Check sheet for the modelled part. Datum: model origin and axes. Units: mm. Face numbers are marked on the shaded views. A direction names the side the tool comes from. Round coordinates to 2 decimals unless told otherwise and drop trailing zeros. Write each loop counter-clockwise with the first axis right and the second up, starting at its lowest first coordinate (ties: lowest second). Pieces come first, ordered by that corner, then holes. Notation, with made-up numbers: (2, -14.5) -> (46, -14.5) arc R24 ccw to (46, 12.5) -> close; hole circle Ø5 at (66.25, 72.5). An arc over 180 degrees is marked (long way). One line per item, written item: value.
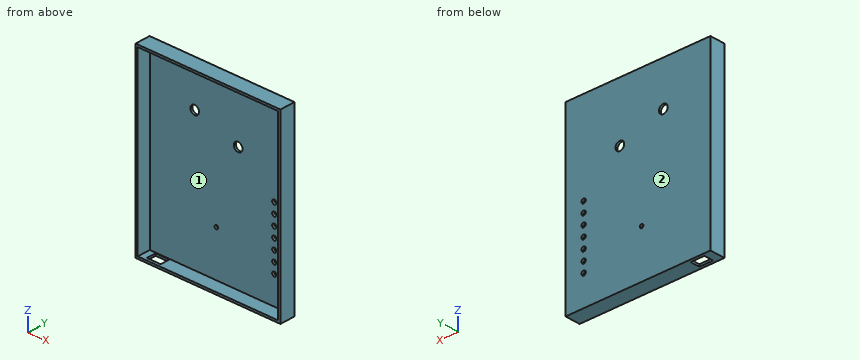
Autodesk Inventor part; units mm, degrees
ref_plane "YZ Plane" through (0, 0, 0) normal (1, 0, 0) x (0, 1, 0)
ref_plane "XZ Plane" through (0, 0, 0) normal (0, 1, 0) x (-1, 0, 0)
ref_plane "XY Plane" through (0, 0, 0) normal (0, 0, 1) x (1, 0, 0)
sketch "block" plane through (0, 0, 0) normal (0, 1, 0) x (-1, 0, 0)
  line L0 (0, 0) -> (-200, 0)
  line L1 (-200, 0) -> (-200, -250)
  line L2 (-200, -250) -> (0, -250)
  line L3 (0, -250) -> (0, 0)
  dimension "d31" = 200
  dimension "d32" = 250
extrude "ext_block" add sketch "block" against normal blind 24
shell "Shell2" thickness 3 removed faces 0
sketch "lines_base" plane through (0, 0, 0) normal (0, 1, 0) x (-1, 0, 0)
  line L0 (0, 0) -> (-200, 0)
  line L1 (-200, 0) -> (-200, -250)
  line L2 (-200, -250) -> (0, -250)
  line L3 (0, -250) -> (0, 0)
  circle A0 centre (-65, -60) radius 6
  circle A1 centre (-125, -80) radius 6
  circle A2 centre (-65, -60) radius 12.5
  circle A3 centre (-65, -60) radius 8.5
  circle A4 centre (-125, -80) radius 8.5
  circle A5 centre (-125, -80) radius 12.5
  circle A6 centre (-175, -125) radius 3
  line L4 (-175, -125) -> (-175, -209)
  line L5 (-175, -125) -> (-91, -125) construction
  circle A7 centre (-175, -139) radius 3
  circle A8 centre (-175, -153) radius 3
  circle A9 centre (-175, -167) radius 3
  circle A10 centre (-175, -181) radius 3
  circle A11 centre (-175, -195) radius 3
  circle A12 centre (-175, -209) radius 3
  circle A13 centre (-95, -185) radius 2.5
  circle A14 centre (-95, -185) radius 5
  point P0 (-200, -125)
  dimension "d0" = 200
  dimension "d1" = 250
  dimension "d2" = 12
  dimension "d3" = 12
  dimension "d4" = 25
  dimension "d5" = 17
  dimension "d6" = 17
  dimension "d7" = 25
  dimension "d8" = 75
  dimension "d9" = 80
  dimension "d10" = 65
  dimension "d11" = 60
  dimension "d12" = 6
  dimension "d13" = 84
  dimension "d14" = 90
  dimension "d15" = 25
  dimension "d16" = 125
  dimension "d19" = 14
  dimension "d24" = 5
  dimension "d25" = 10
  dimension "d26" = 65
  dimension "d27" = 95
extrude "holes" cut sketch "lines_base" against normal up to surface (3 mm away) contours A0 | A1 | A6 | A7 L4 | L4 A7 | A8 L4 | L4 A8 | A9 L4 | L4 A9 | A10 L4 | L4 A10 | A11 L4 | L4 A11 | A12 | A13
sketch "Sketch4" plane through (200, 0, -250) normal (0, 0, -1) x (-1, 0, 0)
  line L0 (188, -4) -> (169, -4)
  line L1 (169, -4) -> (169, -17)
  line L2 (169, -17) -> (188, -17)
  line L3 (188, -17) -> (188, -4)
  line L4 (0, 0) -> (200, 0)
  line L5 (200, 0) -> (200, -24)
  dimension "d40" = 19
  dimension "d41" = 13
  dimension "d42" = 4
  dimension "d43" = 12
extrude "pwr_button_hole" cut sketch "Sketch4" against normal up to surface (3 mm away)
ref_plane "Work Plane1" through (7, -21, -243) normal (0, 1, 0) x (1, 0, 0)
sketch "Sketch5" plane through (7, -21, -243) normal (0, 1, 0) x (1, 0, 0)
  line L0 (-20.9366, 21.7948) -> (229.9216, 21.7948)
  line L1 (229.9216, 21.7948) -> (229.9216, -260.9184)
  line L2 (229.9216, -260.9184) -> (-20.9366, -260.9184)
  line L3 (-20.9366, -260.9184) -> (-20.9366, 21.7948)
  point P0 (-7, -243)
extrude "back_cover_cut" cut sketch "Sketch5" against normal through all
properties part number "back" material "Glass"
Item 1: Thickness scan on line 1 (X direction, y = -5, z = -141); line 2 (Z direction, x = 23, y = -19); line 3 (X direction, y = -1.4, z = -185). Record the ranges inside material, lowest first.
Answer:
line 1: x = 0 to 3, 197 to 200
line 2: z = -250 to -247, -3 to 0
line 3: x = 0 to 92.5, 97.5 to 200
Item 2: Sectioned sample at A-A on z = -60. Enter the section's corners in (x, y).
Answer:
outline: (0, -21) -> (3, -21) -> (3, -3) -> (59, -3) -> (59, 0) -> (0, 0) -> close; (71, -3) -> (197, -3) -> (197, -21) -> (200, -21) -> (200, 0) -> (71, 0) -> close
Item 3: Tool access check on the marked faces 1 and 2. Record the directions out of +Z, -Z, +X, -X, +Y, -Y that give a thin tool (end or side, any length) a straight path to the whole face; none if there is none.
Answer:
face 1: -Y
face 2: +Z, -Z, +X, -X, +Y
Item 4: Sectioned sample at B-B on x = 125. Enter the section's corners in (y, z).
Answer:
outline: (-21, -250) -> (0, -250) -> (0, -86) -> (-3, -86) -> (-3, -247) -> (-21, -247) -> close; (-21, -3) -> (-3, -3) -> (-3, -74) -> (0, -74) -> (0, 0) -> (-21, 0) -> close
Item 5: Depth check by flat-ended pin: P1, Ø14, axis at x = 125, z = -80, coming from the -Y side. Enter the tip coordinate at first touch or a pass-through.
Answer:
P1: stops at y = -3
Item 6: Sectioned sample at C-C on x = 164.5. Enter the section's corners in (y, z), and give its area (3 significant figures).
Answer:
outline: (-21, -250) -> (0, -250) -> (0, 0) -> (-21, 0) -> (-21, -3) -> (-3, -3) -> (-3, -247) -> (-21, -247) -> close
area: 858 mm^2
